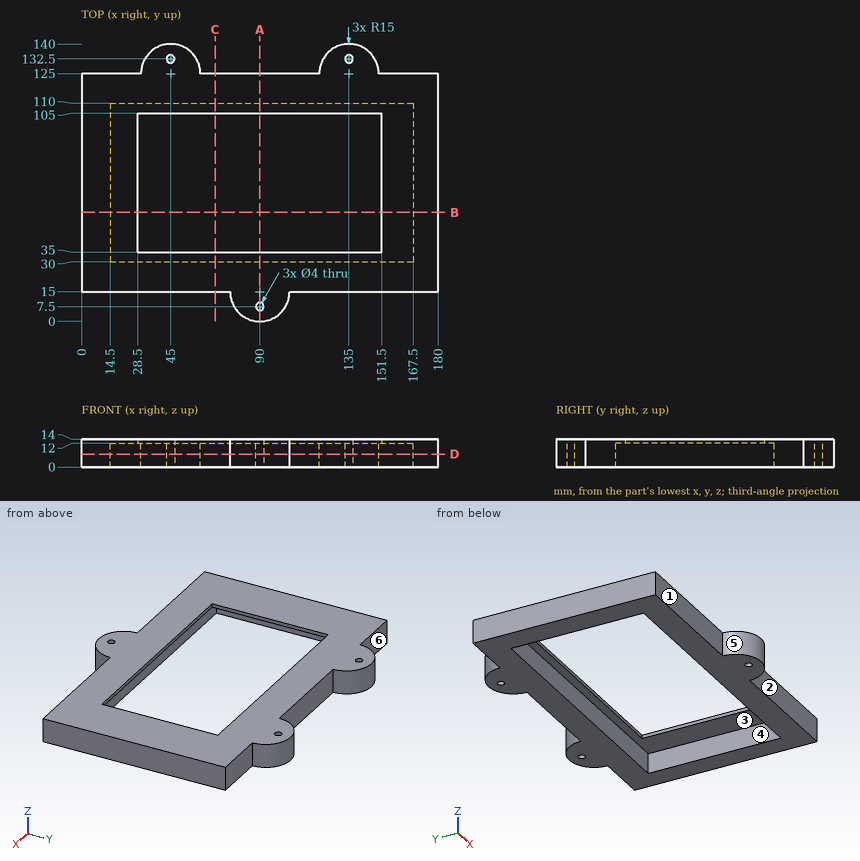
The drawing under review shows one solid part. Ordinate dimensions are in mm from its lowest x, y, z. A direction names the side the tool comes from. Round coordinates to 2 decimals unless told otherwise and drop trailing zeros. Write each loop counter-clockwise with the first axis right and the second up, starting at its lowest first coordinate (ties: lowest second). Pieces come first, ordered by that corner, then holes. Notation, with made-up numbers: (32, 58) - (90, 58) arc R15 ccw to (90, 64) - close; hole circle Ø11 at (41, -38.5). An arc over 180 degrees is marked (long way). Use one line per item in the form item = value.
Q1. Consider section C-C (x = 67.5). State the section outline as (y, z) points.
Answer key:
outline = (15, 0) - (30, 0) - (30, 12) - (35, 12) - (35, 14) - (15, 14) - close; (105, 12) - (110, 12) - (110, 0) - (125, 0) - (125, 14) - (105, 14) - close
Q2. Consider section B-B (y = 55). State the section outline as (x, z) points.
Answer key:
outline = (0, 0) - (14.5, 0) - (14.5, 12) - (28.5, 12) - (28.5, 14) - (0, 14) - close; (151.5, 12) - (167.5, 12) - (167.5, 0) - (180, 0) - (180, 14) - (151.5, 14) - close
Q3. For line 1 (Y direction, x = 135, z = 8); line 2 (Y direction, x = 15, z = 3); line 3 (X direction, y = 132.5, z = 6), list the stretches that pass through material, from the lowest coordinate up. Write a range as [from, to].
Answer key:
line_1 = [15, 30], [110, 130.5], [134.5, 140]
line_2 = [15, 30], [110, 125]
line_3 = [32.01, 43], [47, 57.99], [122.01, 133], [137, 147.99]
Q4. Insertion check: pin 1 Ø7 at (x, z) = (23.5, 4) entering from -Y; pin 2 Ø3 at (x, y) = (90, 7.5) entering from +Z; pin 3 Ø4 at (x, z) = (79, 11) entering from -Y; pin 4 Ø3 at (x, z) = (96, 6.5) entering from -Y. Each pin has a flat end and moves straight along its axis. Give the tip position at first contact, or say it passes through.
Answer key:
pin_1 = 15
pin_2 = through
pin_3 = 3
pin_4 = 0.69
Q5. Consider section A-A (x = 90). State the section outline as (y, z) points, and give its area (3 significant figures).
Answer key:
outline = (0, 0) - (5.5, 0) - (5.5, 14) - (0, 14) - close; (9.5, 0) - (30, 0) - (30, 12) - (35, 12) - (35, 14) - (9.5, 14) - close; (105, 12) - (110, 12) - (110, 0) - (125, 0) - (125, 14) - (105, 14) - close
area = 594 mm2
Q6. Draft analysis for pull direction X (two halves, no side actions). For the marked faces 4, 5 and 6, state which applies: +X half, -X half, draft (parallel to the pull), parting line (faces both ways), or undercut.
Answer key:
face_4 = undercut
face_5 = parting line
face_6 = draft
Q7. Tool access review of the marked faces 1, 2 and 3: name each direction out of +Z, -Z, +X, -X, +Y, -Y from which nothing blocks a thin tool from reaching the whole face with its end or side.
Answer key:
face_1 = +Z, -Z, -X, -Y
face_2 = +Z, -Z, +X, -Y
face_3 = -Z
Q8. Consider section D-D (z = 6.5). State the section outline as (x, y) points.
Answer key:
outline = (0, 15) - (75, 15) arc R15 ccw to (105, 15) - (180, 15) - (180, 125) - (150, 125) arc R15 ccw to (120, 125) - (60, 125) arc R15 ccw to (30, 125) - (0, 125) - close; hole (14.5, 30) - (167.5, 30) - (167.5, 110) - (14.5, 110) - close; hole circle Ø4 at (45, 132.5); hole circle Ø4 at (90, 7.5); hole circle Ø4 at (135, 132.5)
